```python
from build123d import *

# Parameters (mm, degrees)
SKETCH1_R           = 54.61
SKETCH1_R_2         = 52.07
BOSS_EXTRUDE1_DEPTH = 25.4
SKETCH3_R           = 1.905
CUT_EXTRUDE1_DEPTH  = 82.299841328
CIRPATTERN1_COUNT   = 2


with BuildPart() as part:
    # Sketch1 → Boss-Extrude1 (new body)
    with BuildSketch(Plane(origin=(0, 0, 0), x_dir=(1, 0, 0), z_dir=(0, 1, 0))):
        with Locations(Location((0, 0, 0), (0, 0, 270))):
            Circle(SKETCH1_R)
        with Locations(Location((0, 0, 0), (0, 0, 270))):
            Circle(SKETCH1_R_2, mode=Mode.SUBTRACT)
    extrude(amount=BOSS_EXTRUDE1_DEPTH)

    # Sketch3 → Cut-Extrude1 (cut, through all)
    with BuildSketch(Plane.XY):
        with Locations(Location((0, 12.328955527, 0), (0, 0, 90.000000049))):
            Circle(SKETCH3_R)
    cut_extrude1 = extrude(amount=CUT_EXTRUDE1_DEPTH, mode=Mode.SUBTRACT)

    # CirPattern1: Cut-Extrude1 ×2 about axis
    cirpattern1_axis = Axis((0, 25.4, 0), (0, 1, 0))
    for i in range(1, CIRPATTERN1_COUNT):
        add(cut_extrude1.rotate(cirpattern1_axis, i * 360 / CIRPATTERN1_COUNT), mode=Mode.SUBTRACT)


solid = part.part
```
Geometry check sheet. Reference: the model listing, model coordinates, mm. Give positions to 0.01 mm unless a question says otherwise; leave off trailing zeros. Order: outer loops, then holes, each group sorted by start corner. A loop starts at its lowest first (then second) coordinate and runs counter-clockwise, first axis right, second up. Notation, with made-up numbers: (81.5, 49.5) - (134.5, 49.5) arc R19 cw to (134.5, 74.5) - close; hole circle Ø4 at (-24, 36.25). An arc over 180 degrees is marked (long way). Answer in a Markdown table with one row per item. Add a question column.
Q1. Cross-section at B-B, the plane x = 0. Enter the section's corners in (y, z), then the cut area to 3 significant figures.
Q2. Gauge pin test, flat ends, axial feed: pin 1 (5 mm diameter, centred on y = 22.5, z = 31, fed in from +X); pin 2 (5 mm diameter, centred on y = 22, z = -35, fed in from -X); pin 3 (3 mm diameter, centred on x = 34.5, y = 13.5, fed in from +Z); pin 4 (6 mm diameter, centred on x = 0, y = 12.33, fed in from +Z). Record the tip position at first contact, or that the pin passes through.
Q3. Mould release check, pull along Y, two halves, no side actions. Record for faces 1 (the flat face through (-20, 25.4, 48.3)), 2 (the flat face through (-20, 0, 48.3)), 3 (the cylindrical face through (-0.7, 14.1, -53.3)): pulls with the +Y half, pulls with the -Y half, needs draft (parallel to the pull), parting line crosses it, or undercut.
Q4. Cross-section at D-D, the plane y = 23. Enter the section's corners in (x, z).
Q5. Material ranges on probe 1 along X at (y, z) = (19.5, 0); probe 2 along X at (y, z) = (8, -12); probe 3 along Z at (x, y) = (-2, 7.5), recorded low to high. Write a range as from..to.
Q6. Cross-section at C-C, the plane x = 48.5. Enter the section's corners in (y, z).
Q7. Cross-section at A-A, the plane z = -1. Enter the section's corners in (x, y), then the cut area to 3 significant figures.
Check values:
| question | item | result |
|---|---|---|
| 1 | outline | (0, -54.61) - (10.42, -54.61) - (10.42, -52.07) - (0, -52.07) - close; (0, 52.07) - (10.42, 52.07) - (10.42, 54.61) - (0, 54.61) - close; (14.23, -54.61) - (25.4, -54.61) - (25.4, -52.07) - (14.23, -52.07) - close; (14.23, 52.07) - (25.4, 52.07) - (25.4, 54.61) - (14.23, 54.61) - close |
| 1 | area | 110 mm^2 |
| 2 | pin 1 | stops at x = 46.58 |
| 2 | pin 2 | stops at x = -43.89 |
| 2 | pin 3 | stops at z = 43.51 |
| 2 | pin 4 | stops at z = 54.61 |
| 3 | face 1 | pulls with the +Y half |
| 3 | face 2 | pulls with the -Y half |
| 3 | face 3 | undercut |
| 4 | outline | circle Ø109.22 at (0, 0); hole circle Ø104.14 at (0, 0) |
| 5 | probe 1 | x = -54.61..-52.07, 52.07..54.61 |
| 5 | probe 2 | x = -53.28..-50.67, 50.67..53.28 |
| 5 | probe 3 | z = -54.57..-52.03, 52.03..54.57 |
| 6 | outline | (0, -25.1) - (25.4, -25.1) - (25.4, -18.95) - (0, -18.95) - close; (0, 18.95) - (25.4, 18.95) - (25.4, 25.1) - (0, 25.1) - close |
| 7 | outline | (-54.6, 0) - (-52.06, 0) - (-52.06, 25.4) - (-54.6, 25.4) - close; (52.06, 0) - (54.6, 0) - (54.6, 25.4) - (52.06, 25.4) - close |
| 7 | area | 129 mm^2 |
